CAD build for the part. Positions are in the model's coordinates, mm. Give positions to 0.01 mm unless a question says otherwise; leave off trailing zeros. Loops run counter-clockwise (first coordinate to the right, second up) from the corner with the lowest first, then second, coordinate; pieces in that order, holes last.
Item 1: Probe probe 1 along X at (y, z) = (5.5, 26); probe 2 along Z at (x, y) = (45, 8.7); probe 3 along Z at (x, y) = (-45, 1.15). List the from-to ranges inside material, lowest first.
Item 2: Saw through at D-D on x = 13. Give the cut face in (y, z).
Item 3: Saw through at A-A on z = 27. Give the cut face in (x, y), plus the area to 3 significant figures.
Item 4: Saw through at C-C on y = 2.75. Give the cut face in (x, z).
Item 5: Saw through at B-B on x = -29.5. Give the cut face in (y, z), plus the area to 3 significant figures.
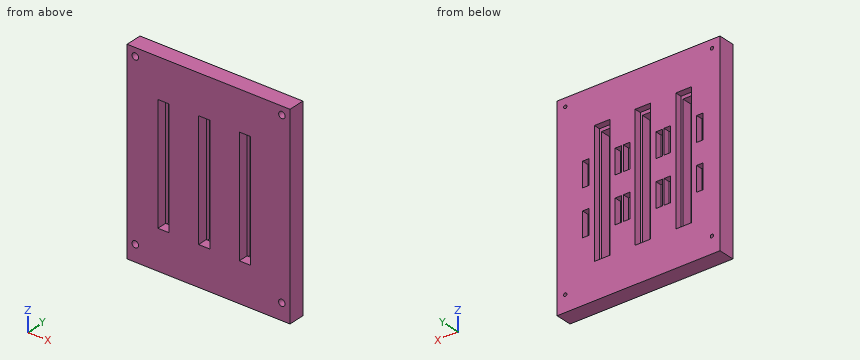
from build123d import *

# Parameters (mm, degrees)
SKETCH2_W           = 100
SKETCH2_H           = 120
SKETCH2_W_2         = 7
SKETCH2_H_2         = 72
BOSS_EXTRUDE1_DEPTH = 10
SKETCH3_W           = 9.5
SKETCH3_H           = 76
SKETCH3_W_2         = 4
SKETCH3_H_2         = 15
CUT_EXTRUDE1_DEPTH  = 4
SKETCH7_R           = 2
CUT_EXTRUDE4_DEPTH  = 5
SKETCH8_R           = 1
CUT_EXTRUDE5_DEPTH  = 5


with BuildPart() as part:
    # Sketch2 → Boss-Extrude1 (new body)
    with BuildSketch(Plane(origin=(0, 0, 0), x_dir=(1, 0, 0), z_dir=(0, 1, 0))):
        Rectangle(SKETCH2_W, SKETCH2_H)
        with Locations((22.353747517, 0)):
            Rectangle(SKETCH2_W_2, SKETCH2_H_2, mode=Mode.SUBTRACT)
        with Locations((-2.646252483, 0)):
            Rectangle(SKETCH2_W_2, SKETCH2_H_2, mode=Mode.SUBTRACT)
        with Locations((-27.646252483, 0)):
            Rectangle(SKETCH2_W_2, SKETCH2_H_2, mode=Mode.SUBTRACT)
    extrude(amount=BOSS_EXTRUDE1_DEPTH)

    # Sketch3 → Cut-Extrude1 (cut)
    with BuildSketch(Plane(origin=(0, 10, 0), x_dir=(1, 0, 0), z_dir=(0, 1, 0))):
        with Locations((-2.646252483, -0.02091915)):
            Rectangle(SKETCH3_W, SKETCH3_H)
        with Locations((-17.646252483, -13.394152505)):
            Rectangle(SKETCH3_W_2, SKETCH3_H_2)
        with Locations((-17.646252483, 14.635235437)):
            Rectangle(SKETCH3_W_2, SKETCH3_H_2)
        with Locations((-37.646252483, 14.635235437)):
            Rectangle(SKETCH3_W_2, SKETCH3_H_2)
        with Locations((-37.646252483, -13.246569784)):
            Rectangle(SKETCH3_W_2, SKETCH3_H_2)
        with Locations((-12.646252483, -13.246569784)):
            Rectangle(SKETCH3_W_2, SKETCH3_H_2)
        with Locations((-12.646252483, 14.635235437)):
            Rectangle(SKETCH3_W_2, SKETCH3_H_2)
        with Locations((7.353747517, 14.635235437)):
            Rectangle(SKETCH3_W_2, SKETCH3_H_2)
        with Locations((12.353747517, 14.635235437)):
            Rectangle(SKETCH3_W_2, SKETCH3_H_2)
        with Locations((12.353747517, -13.246569784)):
            Rectangle(SKETCH3_W_2, SKETCH3_H_2)
        with Locations((7.353747517, -13.246569784)):
            Rectangle(SKETCH3_W_2, SKETCH3_H_2)
        with Locations((32.353747517, -13.246569784)):
            Rectangle(SKETCH3_W_2, SKETCH3_H_2)
        with Locations((32.353747517, 14.635235437)):
            Rectangle(SKETCH3_W_2, SKETCH3_H_2)
        with Locations((-27.646252483, -0.02091915)):
            Rectangle(SKETCH3_W, SKETCH3_H)
        with Locations((22.353747517, -0.02091915)):
            Rectangle(SKETCH3_W, SKETCH3_H)
    extrude(amount=-CUT_EXTRUDE1_DEPTH, mode=Mode.SUBTRACT)

    # Sketch7 → Cut-Extrude4 (cut)
    with BuildSketch(Plane.XZ):
        with Locations((45, -50)):
            Circle(SKETCH7_R)
        with Locations((-45, -50)):
            Circle(SKETCH7_R)
        with Locations((-45, 55)):
            Circle(SKETCH7_R)
        with Locations((45, 55)):
            Circle(SKETCH7_R)
    extrude(amount=-CUT_EXTRUDE4_DEPTH, mode=Mode.SUBTRACT)

    # Sketch8 → Cut-Extrude5 (cut)
    with BuildSketch(Plane(origin=(0, 5, 0), x_dir=(-1, 0, 0), z_dir=(0, -1, 0))):
        with Locations((-45, 50)):
            Circle(SKETCH8_R)
        with Locations((45, 50)):
            Circle(SKETCH8_R)
        with Locations((45, -55)):
            Circle(SKETCH8_R)
        with Locations((-45, -55)):
            Circle(SKETCH8_R)
    extrude(amount=-CUT_EXTRUDE5_DEPTH, mode=Mode.SUBTRACT)


solid = part.part
Results below:
1. probe 1: x = -50 to -31.15, -24.15 to -6.15, 0.85 to 18.85, 25.85 to 50
1. probe 2: z = -60 to -51, -49 to 54, 56 to 60
1. probe 3: z = -60 to -52, -48 to 53, 57 to 60
2. outline: (0, -60) - (10, -60) - (10, -22.14) - (6, -22.14) - (6, -7.14) - (10, -7.14) - (10, 5.75) - (6, 5.75) - (6, 20.75) - (10, 20.75) - (10, 60) - (0, 60) - close
3. outline: (-50, 0) - (-31.15, 0) - (-31.15, 6) - (-32.4, 6) - (-32.4, 10) - (-50, 10) - close; (-24.15, 0) - (-6.15, 0) - (-6.15, 6) - (-7.4, 6) - (-7.4, 10) - (-22.9, 10) - (-22.9, 6) - (-24.15, 6) - close; (0.85, 0) - (18.85, 0) - (18.85, 6) - (17.6, 6) - (17.6, 10) - (2.1, 10) - (2.1, 6) - (0.85, 6) - close; (25.85, 0) - (50, 0) - (50, 10) - (27.1, 10) - (27.1, 6) - (25.85, 6) - close
3. area: 760 mm2
4. outline: (-50, -60) - (50, -60) - (50, 60) - (-50, 60) - close; hole circle Ø4 at (-45, -50); hole circle Ø4 at (-45, 55); hole (-31.15, -36) - (-24.15, -36) - (-24.15, 36) - (-31.15, 36) - close; hole (-6.15, -36) - (0.85, -36) - (0.85, 36) - (-6.15, 36) - close; hole (18.85, -36) - (25.85, -36) - (25.85, 36) - (18.85, 36) - close; hole circle Ø4 at (45, -50); hole circle Ø4 at (45, 55)
5. outline: (0, -60) - (10, -60) - (10, -37.98) - (6, -37.98) - (6, -36) - (0, -36) - close; (0, 36) - (6, 36) - (6, 38.02) - (10, 38.02) - (10, 60) - (0, 60) - close
5. area: 464 mm2
